Design review of the part built by this model. Coordinates are the model's own, in mm. A direction names the side the tool comes from. Coordinates: 2 decimals unless noted, no trailing zeros. Order: outer loops, then holes, each group sorted by start corner. A loop starts at its lowest first (then second) coordinate and runs counter-clockwise, first axis right, second up. Notation, with made-up numbers: (28.25, 79.25) -> (65.25, 79.25) arc R26 cw to (65.25, 107.25) -> close; hole circle Ø9 at (71.25, 32.5). An arc over 180 degrees is marked (long way). Write item = value, one per line.
```python
from build123d import *

# Parameters (mm, degrees)
BOSS_EXTRUDE1_DEPTH = 52
SKETCH2_W           = 30
SKETCH2_H           = 87.134992814
BOSS_EXTRUDE2_DEPTH = 5
SKETCH3_W           = 80
SKETCH3_H           = 30
BOSS_EXTRUDE3_DEPTH = 5
BOSS_EXTRUDE4_DEPTH = 5
CUT_EXTRUDE2_DEPTH  = 5
SKETCH7_R           = 1.75
CUT_EXTRUDE3_DEPTH  = 162.300960939
SKETCH8_W           = 10
SKETCH8_H           = 6
SKETCH8_W_2         = 6
SKETCH8_H_2         = 10
CUT_EXTRUDE4_DEPTH  = 162.300960939


with BuildPart() as part:
    # Sketch1 → Boss-Extrude1 (new body)
    with BuildSketch(Plane(origin=(0, 0, 0), x_dir=(1, 0, 0), z_dir=(0, 1, 0))):
        Polygon((0, 0), (0, 100), (3, 100), (3, 3), (83, 3), (83, 100), (86, 100), (86, 0), align=None)
    extrude(amount=BOSS_EXTRUDE1_DEPTH)

    # Sketch2 → Boss-Extrude2 (add)
    with BuildSketch(Plane(origin=(0, 52, 0), x_dir=(1, 0, 0), z_dir=(0, 1, 0))):
        with Locations((98, 56.432503593)):
            Rectangle(SKETCH2_W, SKETCH2_H)
        with Locations((-12, 56.432503593)):
            Rectangle(SKETCH2_W, SKETCH2_H)
    extrude(amount=BOSS_EXTRUDE2_DEPTH)

    # Sketch3 → Boss-Extrude3 (add)
    with BuildSketch(Plane(origin=(0, 57, 0), x_dir=(1, 0, 0), z_dir=(0, 1, 0))):
        with Locations((43, 85)):
            Rectangle(SKETCH3_W, SKETCH3_H)
    extrude(amount=-BOSS_EXTRUDE3_DEPTH)

    # Sketch5 → Boss-Extrude4 (add)
    with BuildSketch(Plane(origin=(0, 52, 0), x_dir=(1, 0, 0), z_dir=(0, 1, 0))):
        Polygon((0, 12.865007186), (0, 0), (86, 0), (86, 12.865007186), (83, 12.865007186), (83, 3), (3, 3), (3, 12.865007186), align=None)
    extrude(amount=BOSS_EXTRUDE4_DEPTH)

    # Sketch6 → Cut-Extrude2 (cut)
    with BuildSketch(Plane.XY):
        with BuildLine():
            Line((19, 0), (67, 0))
            ThreePointArc((67, 0), (43, 24), (19, 0))
        make_face()
    extrude(amount=-CUT_EXTRUDE2_DEPTH, mode=Mode.SUBTRACT)

    # Sketch7 → Cut-Extrude3 (cut, through all)
    with BuildSketch(Plane(origin=(0, 57, 0), x_dir=(1, 0, 0), z_dir=(0, 1, 0))):
        with Locations(Location((-13.149809764, 22.865007186, 0), (0, 0, 270))):
            Circle(SKETCH7_R)
        with Locations(Location((63, 85, 0), (0, 0, 270))):
            Circle(SKETCH7_R)
        with Locations(Location((98, 22.865007186, 0), (0, 0, 270))):
            Circle(SKETCH7_R)
    extrude(amount=-CUT_EXTRUDE3_DEPTH, mode=Mode.SUBTRACT)

    # Sketch8 → Cut-Extrude4 (cut, through all)
    with BuildSketch(Plane(origin=(0, 57, 0), x_dir=(1, 0, 0), z_dir=(0, 1, 0))):
        with Locations((98, 52.5)):
            Rectangle(SKETCH8_W, SKETCH8_H)
        with Locations((35.5, 85)):
            Rectangle(SKETCH8_W_2, SKETCH8_H_2)
    extrude(amount=-CUT_EXTRUDE4_DEPTH, mode=Mode.SUBTRACT)


solid = part.part
```
(1) We need section D-D (z = -64.5). Write out the cut boundary in (x, y).
Report:
outline = (-27, 52) -> (0, 52) -> (0, 0) -> (3, 0) -> (3, 57) -> (-27, 57) -> close; (83, 0) -> (86, 0) -> (86, 52) -> (113, 52) -> (113, 57) -> (83, 57) -> close
(2) We need section A-A (z = -85). Write out the cut boundary in (x, y), and give its area (4 significant figures).
Report:
outline = (-27, 52) -> (0, 52) -> (0, 0) -> (3, 0) -> (3, 52) -> (32.5, 52) -> (32.5, 57) -> (-27, 57) -> close; (38.5, 52) -> (61.25, 52) -> (61.25, 57) -> (38.5, 57) -> close; (64.75, 52) -> (83, 52) -> (83, 0) -> (86, 0) -> (86, 52) -> (113, 52) -> (113, 57) -> (64.75, 57) -> close
area = 964.5 mm²
(3) Insertion check: pin 1 (13.5 mm diameter, centred on x = -18, z = -40, fed in from -Y); pin 2 (1.5 mm diameter, centred on x = 17.5, y = 45, fed in from +Z); pin 3 (4 mm diameter, centred on y = 11.5, z = -64.5, fed in from -X); pin 4 (5 mm diameter, centred on y = 39.5, z = -67.5, fed in from +X). Each pin has a flat end and moves straight along its axis. Give the tip position at first contact, or say it passes through.
Report:
pin_1 = 52
pin_2 = 0
pin_3 = 0
pin_4 = 86
(4) The part is to be moulded in two halves that separate along Z. For faces 3 (the flat face through (42, 34, 0)), 4 (the flat face through (38.5, 55, -85)), 5 (the flat face through (99, 52, -57)), 6 (the flat face through (35, 55, -80)), say which applies: released by +Z, released by -Z, zero draft, split by the parting line, or undercut.
Report:
face_3 = released by +Z
face_4 = undercut
face_5 = zero draft
face_6 = undercut
(5) For faces 1 (the flat face through (103, 55, -52)), 2 (the flat face through (113, 54, -56)), list the 3-axis set-ups (+Z, -Z, +X, -X, +Y, -Y) from which the entire face can be reached by the end or side of a thin tool; tool diameter is ignored.
Report:
face_1 = +Y, -Y
face_2 = +Z, -Z, +X, +Y, -Y
(6) We need section B-B (x = 43). Write out the cut boundary in (y, z).
Report:
outline = (24, -3) -> (57, -3) -> (57, 0) -> (24, 0) -> close; (52, -100) -> (57, -100) -> (57, -70) -> (52, -70) -> close
(7) We need section C-C (y = 27). Write out the cut boundary in (x, z).
Report:
outline = (0, -100) -> (3, -100) -> (3, -3) -> (83, -3) -> (83, -100) -> (86, -100) -> (86, 0) -> (0, 0) -> close
(8) For L1, parallel to Z at x = 98, y = 53 (3 decimals); L2, parallel to X at y = 7, z = -68.5; L3, parallel to Y at x = 52, z = -79.5, list the stretches that pass through material, from the lowest coordinate up.
Report:
L1 = -100 to -55.5, -49.5 to -24.615, -21.115 to -12.865
L2 = 0 to 3, 83 to 86
L3 = 52 to 57
